```python
from build123d import *

# Parameters (mm, degrees)
ESTRUSIONE1_DEPTH      = 3.495
ESTRUSIONE1_DEPTH_BACK = 3.495
SCHIZZO1_R             = 7.5
SMUSSO1_SIZE           = 0.2
SMUSSO1_SIZE_2         = 0.14484006


with BuildPart() as part:
    # Schizzo1 → Estrusione1 (new, two sides: drawn at the far end of the back side and taken through both)
    with BuildSketch(Plane.XY.offset(-ESTRUSIONE1_DEPTH_BACK)):
        Circle(SCHIZZO1_R)
    extrude(amount=ESTRUSIONE1_DEPTH + ESTRUSIONE1_DEPTH_BACK)

    # Schizzo2 → Taglia-Rivoluzione1 (revolve, cut)
    with BuildSketch(Plane(origin=(0, 0, 0), x_dir=(1, 0, 0), z_dir=(0, 1, 0))):
        with BuildLine():
            Line((0, 6.5), (0, -6.5))
            ThreePointArc((0, -6.5), (-6.5, 0), (0, 6.5))
        make_face()
    revolve(axis=Axis((0, 0, -4.815448708), (0, 0, 1)), mode=Mode.SUBTRACT)

    # Smusso1
    # the kernel refuses this chamfer: 0.2, 0.14484006 mm, written as the material it takes off along each edge
    with BuildSketch(Plane(origin=(0, 0, -3.495), x_dir=(1, 0, 0), z_dir=(0, -1, 0))) as smusso1_piece_1:
        Polygon((7.5, SMUSSO1_SIZE), (7.5 - SMUSSO1_SIZE, 0), (7.5, 0), align=None)
    revolve(axis=Axis((0, 0, -3.495), (0, 0, 1)), mode=Mode.SUBTRACT)
    with BuildSketch(Plane(origin=(0, 0, 3.495), x_dir=(1, 0, 0), z_dir=(0, -1, 0))) as smusso1_piece_2:
        Polygon((7.5, -SMUSSO1_SIZE), (7.5 - SMUSSO1_SIZE, 0), (7.5, 0), align=None)
    revolve(axis=Axis((0, 0, 3.495), (0, 0, 1)), mode=Mode.SUBTRACT)
    with BuildSketch(Plane(origin=(0, 0, 3.495), x_dir=(-1, 0, 0), z_dir=(0, -1, 0))) as smusso1_piece_3:
        with BuildLine():
            Line((5.480417411 + SMUSSO1_SIZE, 0), (5.557122182, 0.12329523))
            ThreePointArc((5.557122182, 0.12329523), (5.519593752, 0.062204519), (5.480417411, 0))
            Line((5.480417411, 0), (5.480417411 + SMUSSO1_SIZE, 0))
        make_face()
    revolve(axis=Axis((0, 0, 3.495), (0, 0, -1)), mode=Mode.SUBTRACT)
    with BuildSketch(Plane(origin=(0, 0, -3.495), x_dir=(-1, 0, 0), z_dir=(0, -1, 0))) as smusso1_piece_4:
        with BuildLine():
            Line((5.480417411 + SMUSSO1_SIZE_2 * 1.00000000281, 0), (5.586985705, -0.173014037))
            ThreePointArc((5.586985705, -0.173014037), (5.535884344, -0.088537827), (5.480417411, 0))
            Line((5.480417411, 0), (5.480417411 + SMUSSO1_SIZE_2 * 1.00000000281, 0))
        make_face()
    revolve(axis=Axis((0, 0, -3.495), (0, 0, -1)), mode=Mode.SUBTRACT)


solid = part.part
```
Read the model definition and answer for the solid it produces. Units are mm, in the model's axes. Coordinates: 2 decimals unless noted, no trailing zeros. Loops run counter-clockwise (first coordinate to the right, second up) from the corner with the lowest first, then second, coordinate; pieces in that order, holes last. Notation, with made-up numbers: (53.5, 61) - (57.5, 61) arc R13 ccw to (57.5, 70) - close; hole circle Ø9 at (66.25, 6). An arc over 180 degrees is marked (long way). Answer in a Markdown table with one row per item.
1. Determine the mould class of faces 1 (the face through (0, -6, 3.495)), 2 (the face through (-7.493, 0.33, -0.046)) for opening direction Y: +Y half, -Y half, draft (parallel to the pull), parting line (faces both ways), or undercut.
Conclusion:
| item | result |
|---|---|
| face 1 | draft |
| face 2 | parting line |
2. Find section B-B, the plane z = 0. Write down the section's boundary in (x, y).
Conclusion:
| item | result |
|---|---|
| outline | circle Ø15 at (0, 0); hole circle Ø13 at (0, 0) |
3. Find section A-A, the plane x = 0. Write down the section's boundary in (y, z) (3 decimals), then the cut area to 3 significant figures.
Conclusion:
| item | result |
|---|---|
| outline | (-7.5, -3.295) - (-7.3, -3.495) - (-5.625, -3.495) - (-5.587, -3.322) arc R6.5 cw to (-5.557, 3.372) - (-5.68, 3.495) - (-7.3, 3.495) - (-7.5, 3.295) - close; (5.557, 3.372) arc R6.5 cw to (5.587, -3.322) - (5.625, -3.495) - (7.3, -3.495) - (7.5, -3.295) - (7.5, 3.295) - (7.3, 3.495) - (5.68, 3.495) - close |
| area | 18.4 mm² |
4. Given pin 1 (1 mm diameter, centred on x = 4.5, z = 0, fed in from -Y); pin 2 (1.5 mm diameter, centred on x = 1.5, z = 2.5, fed in from -Y), each flat-ended and moving along its own axis, determine where each tip first touches the part or whether it passes through.
Conclusion:
| item | result |
|---|---|
| pin 1 | stops at y = -6.34 |
| pin 2 | stops at y = -7.46 |
5. Straight lines are drawn through the part: line 1 (Z direction, x = -5.75, y = 1) (3 decimals); line 2 (Y direction, x = -3, z = -2.5); line 3 (X direction, y = 3.75, z = -0.75). For each, find the intervals that lie inside material, in ascending order.
Conclusion:
| item | result |
|---|---|
| line 1 | z = -3.495 to -2.861, 2.861 to 3.495 |
| line 2 | y = -6.87 to -5.2, 5.2 to 6.87 |
| line 3 | x = -6.5 to -5.26, 5.26 to 6.5 |
6. Find section D-D, the plane z = 1.25. Write down the section's boundary in (x, y).
Conclusion:
| item | result |
|---|---|
| outline | circle Ø15 at (0, 0); hole circle Ø12.76 at (0, 0) |
